```python
from build123d import *

# Parameters (mm, degrees)
BOSS_EXTRUDE1_DEPTH = 9.525
BOSS_EXTRUDE2_DEPTH = 9.525
SKETCH3_R           = 9.525
CUT_EXTRUDE6_DEPTH  = 587.481888574
FILLET1_R           = 15.875


with BuildPart() as part:
    # Sketch1 → Boss-Extrude1 (new body)
    with BuildSketch(Plane(origin=(0, 0, 0), x_dir=(1, 0, 0), z_dir=(0, 1, 0))):
        Polygon((461.512355724, 17.636671785), (558.8, 99.270698215), (558.8, 177.8), (228.6, 177.8), (228.6, -177.8), align=None)
    extrude(amount=BOSS_EXTRUDE1_DEPTH)

    # Sketch1_4 → Boss-Extrude2 (add)
    with BuildSketch(Plane(origin=(0, 0, 0), x_dir=(1, 0, 0), z_dir=(0, 1, 0))):
        Polygon((558.8, -177.8), (558.8, 99.270698215), (461.512355724, 17.636671785), (228.6, -177.8), align=None)
    extrude(amount=BOSS_EXTRUDE2_DEPTH)

    # Sketch3 → Cut-Extrude6 (cut, through all)
    with BuildSketch(Plane.XZ):
        with Locations(Location((393.7, 0, 0), (0, 0, 270))):
            Circle(SKETCH3_R)
        with Locations(Location((311.15, 88.9, 0), (0, 0, 270))):
            Circle(SKETCH3_R)
        with Locations(Location((434.975, 88.9, 0), (0, 0, 270))):
            Circle(SKETCH3_R)
        with Locations(Location((352.425, -88.9, 0), (0, 0, 270))):
            Circle(SKETCH3_R)
    extrude(amount=-CUT_EXTRUDE6_DEPTH, mode=Mode.SUBTRACT)

    # Fillet1
    fillet1_edges = [part.edges().sort_by_distance(p)[0] for p in [
        (228.6, 4.7625, -177.8),
        (228.6, 4.7625, 177.8),
    ]]
    fillet(fillet1_edges, radius=FILLET1_R)


solid = part.part
```
Here's how the part is built. I have some questions about the finished solid (model axes, mm). Coordinates: 2 decimals unless noted, no trailing zeros. Order: outer loops, then holes, each group sorted by start corner. A loop starts at its lowest first (then second) coordinate and runs counter-clockwise, first axis right, second up.
Item 1: If we section it at B-B, the plane x = 311.15: List the corners of the cut face in (y, z) for me (3 decimals), then the cut area to 3 significant figures.
Response values:
outline: (0, -177.8) - (9.525, -177.8) - (9.525, 79.375) - (0, 79.375) - close; (0, 98.425) - (9.525, 98.425) - (9.525, 177.8) - (0, 177.8) - close
area: 3,210 mm2
Item 2: I'm going to push a flat-ended pin straight in: pin 1 Ø22 at (x, z) = (393.7, 0) entering from -Y. Where does the tip first touch, or does it pass through?
Response values:
pin 1: stops at y = 0
Item 3: I need wall thicknesses on probe 1 along X at (y, z) = (7, 88.9) (3 decimals); probe 2 along X at (y, z) = (7, -88.9); probe 3 along X at (y, z) = (3.25, 88). Which ranges of each line are inside material? Lowest first, please.
Response values:
probe 1: x = 228.6 to 301.625, 320.675 to 425.45, 444.5 to 558.8
probe 2: x = 228.6 to 342.9, 361.95 to 558.8
probe 3: x = 228.6 to 301.67, 320.63 to 425.49, 444.46 to 558.8
Item 4: If we section it at A-A, the plane z = 0: List the corners of the cut face in (x, y) for me (3 decimals), then the cut area to 3 significant figures.
Response values:
outline: (228.6, 0) - (384.175, 0) - (384.175, 9.525) - (228.6, 9.525) - close; (403.225, 0) - (558.8, 0) - (558.8, 9.525) - (403.225, 9.525) - close
area: 2,960 mm2
Item 5: Thinking about a two-plate mould opening in X: for faces 1 (the face through (233.4, 4.8, -173.3)), 2 (the face through (404, 5, -177.8)), 3 (the face through (343.127, 4.696, -86.835)), 4 (the face through (444.42, 4.7, 90.14)), which applies, pulls with the +X half, pulls with the -X half, needs draft (parallel to the pull), parting line crosses it, or undercut?
Response values:
face 1: pulls with the -X half
face 2: needs draft
face 3: undercut
face 4: undercut
